Autodesk Fusion 360 part; units mm, degrees
sketch "Sketch1" plane through (0, 0, 0) normal (0, 1, 0) x (1, 0, 0)
  line L0 (-22.5578, -5) -> (57.4422, -5)
  line L1 (57.4422, -5) -> (57.4422, 0)
  line L2 (57.4422, 0) -> (-22.5578, 0)
  line L3 (-22.5578, 0) -> (-22.5578, -5)
  line L4 (14.9422, -5) -> (19.9422, -5)
  line L5 (19.9422, -5) -> (19.9422, -1)
  line L6 (19.9422, -1) -> (14.9422, -1)
  line L7 (14.9422, -1) -> (14.9422, -5)
  dimension "d1" = 5
  dimension "d2" = 80
  dimension "d3" = 5
  dimension "d4" = 4
  dimension "d5" = 37.5
extrude "Extrude1" add sketch "Sketch1" along normal blind 40 contours L0 L1 L2 L3 L5 L6 L7
fillet "Fillet1" radius 2 1 edges at (57.4422, 20, 5)
fillet "Fillet2" radius 2 1 edges at (-22.5578, 20, 5)
fillet "Fillet3" radius 2 3 edges at (-22.5578, 0, 1.5) (-21.972, 0, 4.4142) (-2.8078, 0, 5)
fillet "Fillet4" radius 2 3 edges at (37.6922, 0, 5) (56.8564, 0, 4.4142) (57.4422, 0, 1.5)
fillet "Fillet5" radius 2 3 edges at (37.6922, 40, 5) (56.8564, 40, 4.4142) (57.4422, 40, 1.5)
fillet "Fillet6" radius 2 3 edges at (-22.5578, 40, 1.5) (-21.972, 40, 4.4142) (-2.8078, 40, 5)
For this review, take the finished solid that the model builds, in its own axes (mm). A direction names the side the tool comes from. Round coordinates to 2 decimals unless told otherwise and drop trailing zeros. Loops run counter-clockwise (first coordinate to the right, second up) from the corner with the lowest first, then second, coordinate; pieces in that order, holes last.
(1) We need section B-B (y = 36). Give the boundary of the cut face in (x, z), plus the area to 3 significant figures.
Returned:
outline: (-22.56, 0) - (57.44, 0) - (57.44, 3) arc R2 ccw to (55.44, 5) - (19.94, 5) - (19.94, 1) - (14.94, 1) - (14.94, 5) - (-20.56, 5) arc R2 ccw to (-22.56, 3) - close
area: 378 mm2
(2) We need section A-A (z = 1.95). Give the boundary of the cut face in (x, y).
Returned:
outline: (-22.56, 2) arc R2 ccw to (-20.56, 0) - (14.94, 0) - (14.94, 40) - (-20.56, 40) arc R2 ccw to (-22.56, 38) - close; (19.94, 0) - (55.44, 0) arc R2 ccw to (57.44, 2) - (57.44, 38) arc R2 ccw to (55.44, 40) - (19.94, 40) - close
(3) Mouldability with a two-part tool opening along X and no side actions: class faces 3 (the flat face through (17, 20, 1)), 4 (the flat face through (16.9, 40, 0.8)), 5 (the cylindrical face through (-21.987, 20.252, 4.399)) as released by +X, released by -X, zero draft, split by the parting line, or undercut.
Returned:
face 3: undercut
face 4: zero draft
face 5: released by -X
(4) Wall thickness on line 1 along X through (y, z) = (16, 2.5); line 2 along Z through (x, y) = (17.5, 26); line 3 along X through (y, z) = (23.5, 3.35): over which ranges is each line inside the solid? List them lowest first.
Returned:
line 1: x = -22.56 to 14.94, 19.94 to 57.44
line 2: z = 0 to 1
line 3: x = -22.53 to 14.94, 19.94 to 57.41
(5) Tool access review of faces 1 (the flat face through (19.942, 20, 3)), 2 (the flat face through (18, 20, 0)): name each direction out of +Z, -Z, +X, -X, +Y, -Y from which nothing blocks a thin tool from reaching the whole face with its end or side.
Returned:
face 1: +Z, +Y, -Y
face 2: -Z, +X, -X, +Y, -Y
(6) Clearance check with a flat-ended pin moving along its axis: P1, Ø2.5, axis at x = 18, y = 12, coming from the +Z side. State where the tip first meets the part, or that it passes through.
Returned:
P1: stops at z = 1
